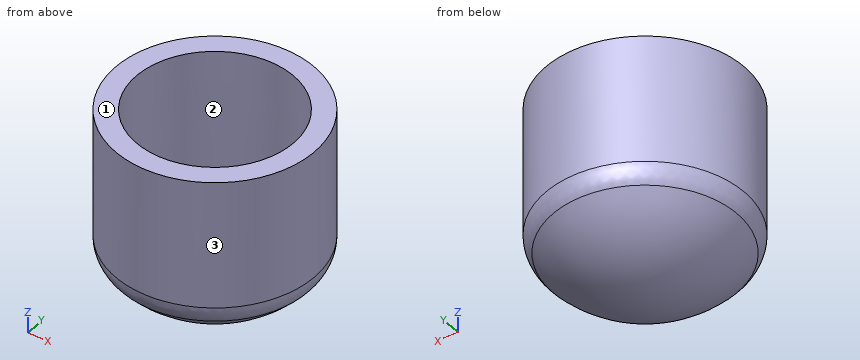
from build123d import *

# Parameters (mm, degrees)
FILLET1_R = 4.826


with BuildPart() as part:
    # Sketch2 → Revolve1 (revolve)
    with BuildSketch(Plane(origin=(0, 0, 0), x_dir=(0, 0, -1), z_dir=(1, 0, 0))):
        with BuildLine():
            Line((-16.0401, -13.4366), (-16.0401, -16.9926))
            Line((-16.0401, -16.9926), (7.50547048, -16.9926))
            ThreePointArc((7.50547048, -16.9926), (13.786577126, -9.507738372), (16.0401, 0))
            Line((16.0401, 0), (12.0523, 0))
            ThreePointArc((12.0523, 0), (10.999645869, -5.924050901), (7.970561543, -11.122811132))
            ThreePointArc((7.970561543, -11.122811132), (6.613783182, -12.155372908), (4.948709843, -12.5222))
            Line((4.948709843, -12.5222), (4.2799, -12.5222))
            Line((4.2799, -12.5222), (4.2799, -13.2842))
            Line((4.2799, -13.2842), (-16.0401, -13.4366))
        make_face()
    revolve(axis=Axis((0, 0, 16.0401), (0, 0, -1)))

    # Fillet1
    fillet1_edges = [part.edges().sort_by_distance(p)[0] for p in [
        (0, 16.9926, -7.50547048),
    ]]
    fillet(fillet1_edges, radius=FILLET1_R)


solid = part.part
Geometry check sheet. Reference: the model listing, model coordinates, mm. Face numbers are marked on the shaded views. Round coordinates to 2 decimals unless told otherwise and drop trailing zeros. Order: outer loops, then holes, each group sorted by start corner. A loop starts at its lowest first (then second) coordinate and runs counter-clockwise, first axis right, second up. Notation, with made-up numbers: M 76.5,82 L 125.5,82 A24 cw 125.5,112 Z; hole C 46.5,66.5 d10. An arc over 180 degrees is marked long. Answer in a Markdown table with one row per item. Add a question column.
Item 1: Draft check along Y on the marked faces 1, 2 and 3. Enter one of: released by +Y, released by -Y, zero draft, split by the parting line, or undercut.
Item 2: Depth check by flat-ended pin: pin 1 Ø8 at (x, z) = (12, 9) entering from -Y; pin 2 Ø2 at (y, z) = (-7, 6.5) entering from -X; pin 3 Ø1 at (x, z) = (-4, -2.5) entering from +Y; pin 4 Ø12 at (y, z) = (1, 2.5) entering from -X. Enter the tip coordinate at first touch or a pass-through.
Item 3: Material ranges on L1, parallel to X at y = 0, z = -4.6; L2, parallel to X at y = 0, z = -4, recorded low to high. Write a range as [from, to].
Item 4: Sectioned sample at A-A, the plane z = 13. Enter the section's corners in (x, y).
Filled in:
| question | item | result |
|---|---|---|
| 1 | face 1 | zero draft |
| 1 | face 2 | undercut |
| 1 | face 3 | split by the parting line |
| 2 | pin 1 | stops at y = -14.99 |
| 2 | pin 2 | stops at x = -15.9 |
| 2 | pin 3 | stops at y = 16.63 |
| 2 | pin 4 | stops at x = -16.99 |
| 3 | L1 | x = [-16.99, -12.52], [12.52, 16.99] |
| 3 | L2 | x = [-16.99, -13.29], [13.29, 16.99] |
| 4 | outline | C 0,0 d33.99; hole C 0,0 d26.83 |
